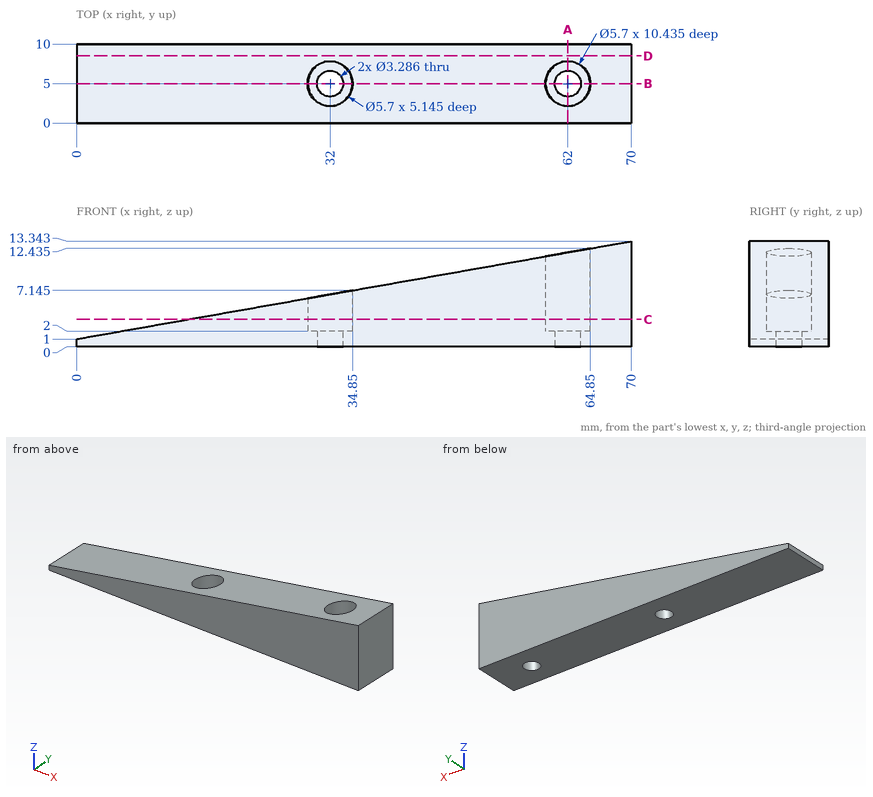
Could you check a few things on this drawing? It's one solid part, dimensions in mm from its lowest x, y, z. Round coordinates to 2 decimals unless told otherwise and drop trailing zeros. Loops run counter-clockwise (first coordinate to the right, second up) from the corner with the lowest first, then second, coordinate; pieces in that order, holes last.
Q1. I want a section at C-C (z = 3.5). Write out the boundary of the cut face in (x, y), and give its area (3 significant figures).
Q2. For P1, Ø4.5, axis at x = 32, y = 5, coming from the -Z side; P2, Ø5, axis at x = 62, y = 5, coming from the +Z side; P3, Ø3, axis at x = 63.5, y = 4.5, coming from the +Z side; P4, Ø6, axis at x = 13.5, z = 8.5, coming from the -Y side, each with a flat end and sliding along its axis, tell me the tip position at first contact or that it passes through.
Q3. I want a section at A-A (x = 62). Write out the boundary of the cut face in (y, z).
Q4. I want a section at B-B (y = 5). Give the number of separate pieces and of enclosed holes in the cut face, and give its area (3 significant figures).
Q5. Please list where these lines run through material, in increasing order: L1, parallel to Y at x = 62, z = 1; L2, parallel to Y at x = 62, z = 8.25; L3, parallel to Z at x = 48, y = 4.5.
Q6. I want a section at D-D (y = 8.5). Write out the boundary of the cut face in (x, z).
Answer below:
1. outline: (14.18, 0) - (70, 0) - (70, 10) - (14.18, 10) - close; hole circle Ø5.7 at (32, 5); hole circle Ø5.7 at (62, 5)
1. area: 507 mm2
2. P1: stops at z = 0
2. P2: stops at z = 2
2. P3: stops at z = 12.46
2. P4: passes through
3. outline: (0, 0) - (3.36, 0) - (3.36, 2) - (2.15, 2) - (2.15, 11.93) - (0, 11.93) - close; (6.64, 0) - (10, 0) - (10, 11.93) - (7.85, 11.93) - (7.85, 2) - (6.64, 2) - close
4. separate pieces: 3
4. enclosed holes: 0
4. area: 406 mm2
5. L1: y = 0 to 3.36, 6.64 to 10
5. L2: y = 0 to 2.15, 7.85 to 10
5. L3: z = 0 to 9.46
6. outline: (0, 0) - (70, 0) - (70, 13.34) - (0, 1) - close
